Here's how the part is built. I have some questions about the finished solid (model axes, mm). A direction names the side the tool comes from. Round coordinates to 2 decimals unless told otherwise and drop trailing zeros. Order: outer loops, then holes, each group sorted by start corner. A loop starts at its lowest first (then second) coordinate and runs counter-clockwise, first axis right, second up. Notation, with made-up numbers: M 8.25,2 L 30.25,2 A14 cw 30.25,17 Z; hole C 38.5,-8 d8. An arc over 180 degrees is marked long. Answer as CSV lines item,"result". Start each with the question number.
```python
from build123d import *

# Parameters (mm, degrees)
F1_DEPTH = 111


with BuildPart() as f1:
    # F0 (on Top) → F1 (new body)
    with BuildSketch(Plane.XY):
        Polygon((6.167513, 15), (6.167513, 0), (21.167513, 0), (21.167513, 27), (-8.832487, 27), (-8.832487, 15), align=None)
        with BuildLine():
            Line((-8.832487, 27), (21.167513, 27))
            ThreePointArc((21.167513, 27), (6.167513, 42), (-8.832487, 27))
        make_face()
    extrude(amount=F1_DEPTH)


solid = f1.part
```
Item 1: If I drill on line 1 along Y through (x, z) = (5.5, 86); line 2 along X through (y, z) = (4.5, 45.5); line 3 along Y through (x, z) = (-0.25, 51), over which ranges is the centre line in solid material (lowest first)?
Item 2: If we section it at A-A on z = 70: Please give me the cut outline in (x, y), and give its area (3 significant figures).
Item 3: If we section it at B-B on y = 4.5: Please give me the cut outline in (x, z), and give its area (4 significant figures).
Item 4: For P1, Ø12, axis at x = 1, z = 74.5, coming from the -Y side; P2, Ø4.5, axis at y = 8, z = 67.5, coming from the -X side; P3, Ø4, axis at x = -3.5, z = 40, coming from the -Y side, each with a flat end and sliding along its axis, tell me the tip position at first contact or that it passes through.
Item 5: Which directions (+Z, -Z, +X, -X, +Y, -Y) give clear straight access to the entire face, cutting with the end or side of a thin tool? Please do faces 1 (the flat face through (6, 21, 0)), 2 (the flat face through (6.168, 8, 55)).
Item 6: If we section it at C-C on x = 3: Please give me the cut outline in (y, z), and give its area (3 significant figures).
Geometry says:
1,line 1,"15 to 41.99"
1,line 2,"6.17 to 21.17"
1,line 3,"15 to 40.56"
2,outline,"M -8.83,15 L 6.17,15 L 6.17,0 L 21.17,0 L 21.17,27 A15 ccw -8.83,27 Z"
2,area,"938 mm²"
3,outline,"M 6.17,0 L 21.17,0 L 21.17,111 L 6.17,111 Z"
3,area,"1,665 mm²"
4,P1,"y = 0"
4,P2,"x = 6.17"
4,P3,"y = 15"
5,face 1,"-Z, +X, -X, +Y, -Y"
5,face 2,"+Z, -Z, -X, -Y"
6,outline,"M 15,0 L 41.66,0 L 41.66,111 L 15,111 Z"
6,area,"2,960 mm²"
